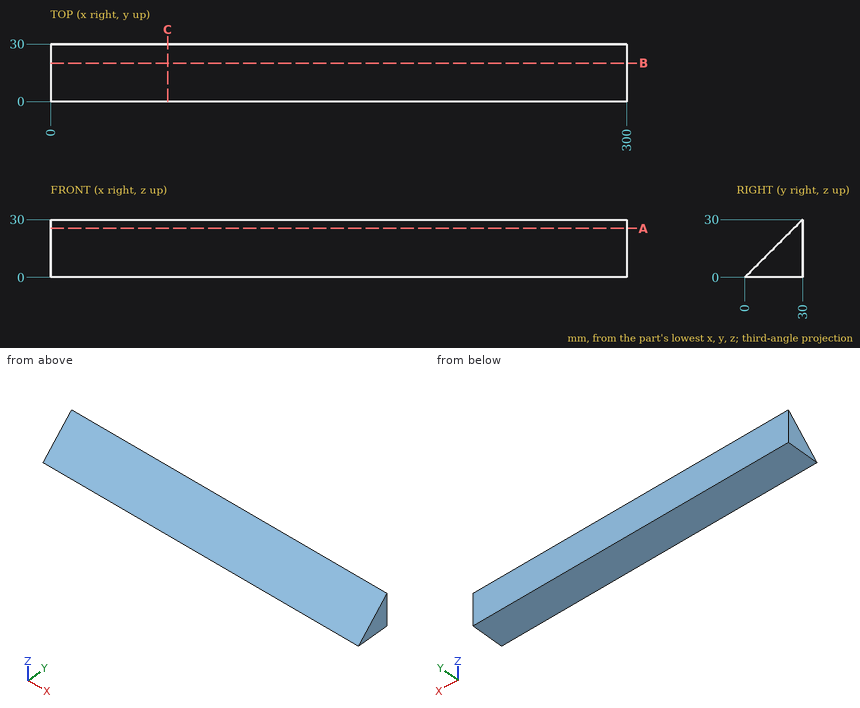
The figure shows three views and two pictorial views of one solid part (mm, origin at its lowest corner). Answer the questions. Give positions to 0.01 mm unless a question says otherwise; leave off trailing zeros. Order: outer loops, then holes, each group sorted by start corner. A loop starts at its lowest first (then second) coordinate and runs counter-clockwise, first axis right, second up. Notation, with made-up numbers: (53, 71.25) -> (88, 71.25) arc R20 cw to (88, 83.25) -> close; hole circle Ø4 at (-16, 79). An arc over 180 degrees is marked (long way). Answer as a JSON object with one key per item and string values. Group by question number.
Item 1: Consider L1, parallel to Y at x = 84, z = 6.5; L2, parallel to Z at x = 130.5, y = 28; L3, parallel to Y at x = 106, z = 7. Determine where each line is inside the solid, lowest interval first. Write a range as from..to.
Item 2: Flat-ended cylindrical pins translate along their axes: pin 1 (6 mm diameter, centred on x = 211.5, y = 5, fed in from +Z); pin 2 (5 mm diameter, centred on y = 21, z = 22, fed in from +X). Find the tip coordinate at first contact, or state that the pin passes through.
Item 3: The part is cut by section A-A on z = 25.5. Write down the section's boundary in (x, y), and give its area (3 significant figures).
Item 4: The part is cut by section B-B on y = 20. Write down the section's boundary in (x, z), and give its area (3 significant figures).
Item 5: The part is cut by section C-C on x = 61. Write down the section's boundary in (y, z), and give its area (3 significant figures).
Result set:
{
 "1": {"L1": "6.5..30", "L2": "0..28", "L3": "7..30"},
 "2": {"pin 1": "z = 8", "pin 2": "x = 300"},
 "3": {"outline": "(0, 25.5) -> (300, 25.5) -> (300, 30) -> (0, 30) -> close", "area": "1,350 mm²"},
 "4": {"outline": "(0, 0) -> (300, 0) -> (300, 20) -> (0, 20) -> close", "area": "6,000 mm²"},
 "5": {"outline": "(0, 0) -> (30, 0) -> (30, 30) -> close", "area": "450 mm²"}
}
